Verification items for the finished model (mm, model axes). A direction names the side the tool comes from. Give positions to 0.01 mm unless a question says otherwise; leave off trailing zeros. Write each loop counter-clockwise with the first axis right and the second up, starting at its lowest first coordinate (ties: lowest second). Pieces come first, ordered by that corner, then holes. Notation, with made-up numbers: M 23,65 L 45,65 A22 ccw 45,75 Z; hole C 15,88.25 d3. An arc over 180 degrees is marked long. Write item = value, one per line.
from build123d import *

# Parameters (mm, degrees)
SKETCH1_R           = 1.75
BOSS_EXTRUDE3_DEPTH = 2
BOSS_EXTRUDE4_DEPTH = 20
BOSS_EXTRUDE5_DEPTH = 4


with BuildPart() as part:
    # Sketch1 → Boss-Extrude3 (new body)
    # profile 1 of 3: a face of its own
    with BuildSketch(Plane(origin=(0, 0, 0), x_dir=(1, 0, 0), z_dir=(0, 1, 0))):
        with BuildLine():
            Line((0.004495957, 4.5), (-2.5, 4.5))
            ThreePointArc((-2.5, 4.5), (-7, 0), (-2.5, -4.5))
            Line((-2.5, -4.5), (0.004495957, -4.5))
            ThreePointArc((0.004495957, -4.5), (2.65, 0), (0.004495957, 4.5))
        make_face()
        with Locations(Location((-2.5, 0, 0), (0, 0, 270))):
            Circle(SKETCH1_R, mode=Mode.SUBTRACT)
    # profile 2 of 3: a face of its own
    with BuildSketch(Plane(origin=(0, 0, 0), x_dir=(1, 0, 0), z_dir=(0, 1, 0))):
        with BuildLine():
            Line((2.508991915, 4.5), (0.004495957, 4.5))
            ThreePointArc((0.004495957, 4.5), (2.65, 0), (0.004495957, -4.5))
            Line((0.004495957, -4.5), (2.508991915, -4.5))
            Line((2.508991915, -4.5), (7, -4.5))
            Line((7, -4.5), (7, 4.5))
            Line((7, 4.5), (2.508991915, 4.5))
        make_face()
        with BuildLine():
            ThreePointArc((4.25, 3), (5, 3.75), (5.75, 3))
            Line((5.75, 3), (5.75, -3))
            ThreePointArc((5.75, -3), (5, -3.75), (4.25, -3))
            Line((4.25, -3), (4.25, 3))
        make_face(mode=Mode.SUBTRACT)
    # profile 3 of 3: a face of its own
    with BuildSketch(Plane(origin=(0, 0, 0), x_dir=(1, 0, 0), z_dir=(0, 1, 0))):
        with BuildLine():
            Line((4.25, 3), (4.25, -3))
            ThreePointArc((4.25, -3), (5, -3.75), (5.75, -3))
            Line((5.75, -3), (5.75, 3))
            ThreePointArc((5.75, 3), (5, 3.75), (4.25, 3))
        make_face()
    extrude(amount=BOSS_EXTRUDE3_DEPTH)

    # Sketch1_3 → Boss-Extrude4 (add)
    with BuildSketch(Plane(origin=(0, 0, 0), x_dir=(1, 0, 0), z_dir=(0, 1, 0))):
        with BuildLine():
            ThreePointArc((0.004495957, 4.5), (2.65, 0), (0.004495957, -4.5))
            Line((0.004495957, -4.5), (7, -4.5))
            Line((7, -4.5), (7, 4.5))
            Line((7, 4.5), (0.004495957, 4.5))
        make_face()
    extrude(amount=-BOSS_EXTRUDE4_DEPTH)

    # Sketch1_5 → Boss-Extrude5 (add)
    with BuildSketch(Plane(origin=(0, 0, 0), x_dir=(1, 0, 0), z_dir=(0, 1, 0))):
        with BuildLine():
            Line((4.25, 3), (4.25, -3))
            ThreePointArc((4.25, -3), (5, -3.75), (5.75, -3))
            Line((5.75, -3), (5.75, 3))
            ThreePointArc((5.75, 3), (5, 3.75), (4.25, 3))
        make_face()
    extrude(amount=BOSS_EXTRUDE5_DEPTH)

    # Mirror1: part across plane


with BuildPart() as part_1:
    add(part.part)
    add(part.part.mirror(Plane.ZX.offset(-20)))


solid = part_1.part
1) Cross-section at C-C on x = 0.5. Record the boundary of the cut face in (y, z).
From the geometry:
outline = M -42,-4.5 L 2,-4.5 L 2,4.5 L -42,4.5 Z; hole M -40,-4.19 L 0,-4.19 L 0,4.19 L -40,4.19 Z
2) Tool access check on faces 1 (the flat face through (-2, -40, 2)), 2 (the flat face through (4.25, 3, 0)), 3 (the flat face through (5.75, -43, 0)), 4 (the flat face through (4.25, -43, 0)). Record the directions out of +Z, -Z, +X, -X, +Y, -Y that give a thin tool (end or side, any length) a straight path to the whole face; none if there is none.
From the geometry:
face_1 = -X
face_2 = +Z, -Z, -X, +Y
face_3 = +Z, -Z, +X, -Y
face_4 = +Z, -Z, -X, -Y
3) Draft check along X on faces 5 (the flat face through (0, 2, 0)), 6 (the cylindrical face through (-7, 1, 0)), 7 (the cylindrical face through (-4.21, 0.99, -0.38)). Enter one of: +X half, -X half, draft (parallel to the pull), parting line (faces both ways), or undercut.
From the geometry:
face_5 = draft
face_6 = -X half
face_7 = undercut
4) Cross-section at A-A on z = 0. Record the boundary of the cut face in (x, y), plus the area to 3 significant figures.
From the geometry:
outline = M -7,-42 L -4.25,-42 L -4.25,-40 L -7,-40 Z; M -7,0 L -4.25,0 L -4.25,2 L -7,2 Z; M -0.75,-42 L 4.25,-42 L 4.25,-44 L 5.75,-44 L 5.75,-42 L 7,-42 L 7,2 L 5.75,2 L 5.75,4 L 4.25,4 L 4.25,2 L -0.75,2 L -0.75,0 L 2.65,0 L 2.65,-40 L -0.75,-40 Z
area = 222 mm^2
5) Depth check by flat-ended pin: P1, Ø1.6, axis at y = 3.5, z = -1.5, coming from the -X side; P2, Ø2.5, axis at x = -1.5, z = -1.5, coming from the -Y side; P3, Ø1, axis at y = -43, z = 1, coming from the +X side. Enter the tip coordinate at first touch or a pass-through.
From the geometry:
P1 = 4.25
P2 = -42
P3 = 5.75
6) Material ranges on probe 1 along X at (y, z) = (1.65, 0); probe 2 along Y at (x, z) = (2.25, 1.25); probe 3 along Y at (x, z) = (4.5, -4), recorded low to high. Write a range as from..to.
From the geometry:
probe_1 = -7..-4.25, -0.75..7
probe_2 = -42..-40, 0..2
probe_3 = -42..2
7) Cross-section at B-B on y = -20. Record the boundary of the cut face in (x, z), plus the area to 3 significant figures.
From the geometry:
outline = M 0,-4.5 L 7,-4.5 L 7,4.5 L 0,4.5 A5.15 cw Z
area = 46.0 mm^2
